Build history of the part. All positions in model axes, mm. Round coordinates to 2 decimals unless told otherwise and drop trailing zeros. Order: outer loops, then holes, each group sorted by start corner. A loop starts at its lowest first (then second) coordinate and runs counter-clockwise, first axis right, second up. Notation, with made-up numbers: M -6,32 L -2,32 A33 ccw -2,67 Z; hole C 10.5,8.25 d11. An arc over 180 degrees is marked long. One line per question, with ' | ' between items. Start each with the question number.
from build123d import *

# Parameters (mm, degrees)
F0_W     = 3.05
F0_H     = 20
F0_W_2   = 20
F0_H_2   = 3.05
F1_DEPTH = 3


with BuildPart() as f1:
    # F0 (on Right) → F1 (new body)
    with BuildSketch(Plane.YZ):
        Polygon((28.35, -45), (42, -45), (42, -28.35), (42, -8.35), (42, 8.35), (42, 28.35), (42, 45), (25.35, 45), (5.35, 45), (-5.35, 45), (-25.35, 45), (-42, 45), (-42, 28.35), (-42, 8.35), (-42, -8.35), (-42, -28.35), (-42, -45), (-28.35, -45), (-8.35, -45), (8.35, -45), align=None)
        with Locations((-43.525, 18.35)):
            Rectangle(F0_W, F0_H)
        with Locations((-43.525, -18.35)):
            Rectangle(F0_W, F0_H)
        with Locations((-18.35, -46.525)):
            Rectangle(F0_W_2, F0_H_2)
        with Locations((18.35, -46.525)):
            Rectangle(F0_W_2, F0_H_2)
        with Locations((43.525, -18.35)):
            Rectangle(F0_W, F0_H)
        with Locations((43.525, 18.35)):
            Rectangle(F0_W, F0_H)
        with Locations((15.35, 46.525)):
            Rectangle(F0_W_2, F0_H_2)
        with Locations((-15.35, 46.525)):
            Rectangle(F0_W_2, F0_H_2)
    extrude(amount=F1_DEPTH)


solid = f1.part
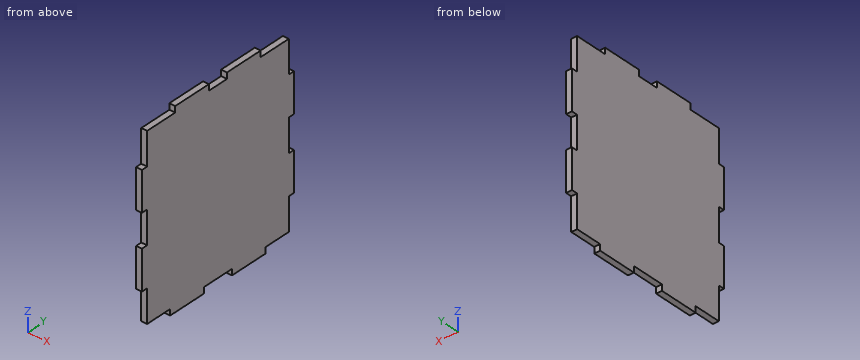
Item 1: Cut at B-B on y = -33. Write the cut outline in (x, z).
Item 2: Flat gauge pins, fed straight in: pin 1 (1 mm diameter, centred on x = 2.5, y = 5, fed in from +Z); pin 2 (1.5 mm diameter, centred on x = 1, y = 0.5, fed in from +Z); pin 3 (1.5 mm diameter, centred on x = 2, y = 44, fed in from +Z); pin 4 (1.5 mm diameter, centred on x = 1, z = 47, fed in from +Y). Where does each tip first touch, or does it go through?
Item 3: Cut at A-A on z = 40.5. Write the cut outline in (x, y), then the cut area to 3 significant figures.
Item 4: Wall check: line 1 along Y through (x, z) = (2.7, -7); line 2 along Z through (x, y) = (2.2, 27); line 3 along Z through (x, y) = (1.4, -6.5). Give the ranges that are in metal, low to high. Write a range as [from, to].
Results found:
1) outline: M 0,-45 L 3,-45 L 3,45 L 0,45 Z
2) pin 1: stops at z = 48.05 | pin 2: stops at z = 45 | pin 3: stops at z = 28.35 | pin 4: stops at y = 25.35
3) outline: M 0,-42 L 3,-42 L 3,42 L 0,42 Z | area: 252 mm^2
4) line 1: y = [-42, 42] | line 2: z = [-48.05, 45] | line 3: z = [-45, 48.05]
